Design review of the part built by this model. Coordinates are the model's own, in mm. A direction names the side the tool comes from. Give positions to 0.01 mm unless a question says otherwise; leave off trailing zeros. Loops run counter-clockwise (first coordinate to the right, second up) from the corner with the lowest first, then second, coordinate; pieces in that order, holes last. Notation, with made-up numbers: M 3.5,65.25 L 17.5,65.25 A13 ccw 17.5,85.25 Z; hole C -9.5,48 d9. An arc over 180 degrees is marked long. Use CSV: the item, a comma, the result in double quotes.
from build123d import *

# Parameters (mm, degrees)
PIPESKETCH_R    = 16.764
PIPESKETCH_R_2  = 13.3858
EXTRUSION_DEPTH = 78.43305879
SKETCH_1_R      = 16.764
SKETCH_1_R_2    = 13.3858
REVOLVE_1_ANGLE = 45.819311821
SKETCH_2_R      = 16.764
SKETCH_2_R_2    = 13.3858
EXTRUDE_1_DEPTH = 197.43866419
SKETCH_3_R      = 16.764
SKETCH_3_R_2    = 13.3858
REVOLVE_2_ANGLE = 90
SKETCH_4_R      = 16.764
SKETCH_4_R_2    = 13.3858
EXTRUDE_2_DEPTH = 120.923725302


with BuildPart() as part:
    # PipeSketch → Extrusion (new body)
    with BuildSketch(Plane.XY):
        Circle(PIPESKETCH_R)
        Circle(PIPESKETCH_R_2, mode=Mode.SUBTRACT)
    extrude(amount=EXTRUSION_DEPTH)

    # 草图1 → 旋转1 (revolve)
    with BuildSketch(Plane.XY.offset(78.43305879)):
        with Locations(Location((0, 0, 0), (0, 0, 40.203758457))):
            Circle(SKETCH_1_R)
        with Locations(Location((0, 0, 0), (0, 0, 40.203758457))):
            Circle(SKETCH_1_R_2, mode=Mode.SUBTRACT)
    revolve(axis=Axis((-29.09901546, -24.593846776, 78.43305879), (0.6455077894006402, -0.7637536866183356, 0)), revolution_arc=REVOLVE_1_ANGLE)

    # 草图2 → 凸台-拉伸1 (add)
    with BuildSketch(Plane(origin=(-44.905078471, -37.952783004, 57.137323745), x_dir=(0.8366600265340762, -0.3030542664308184, 0.4562434784170373), z_dir=(-0.5477225575051652, -0.4629230385328477, 0.6969234250586765))):
        with Locations(Location((43.130838557, 52.305939514, 0), (0, 0, 50.491424948))):
            Circle(SKETCH_2_R)
        with Locations(Location((43.130838557, 52.305939514, 0), (0, 0, 50.491424948))):
            Circle(SKETCH_2_R_2, mode=Mode.SUBTRACT)
    extrude(amount=EXTRUDE_1_DEPTH)

    # 草图3 → 旋转2 (revolve)
    with BuildSketch(Plane(origin=(-153.046688572, -129.351689355, 194.736953831), x_dir=(0.8366600265340762, -0.3030542664308184, 0.4562434784170373), z_dir=(-0.5477225575051652, -0.4629230385328477, 0.6969234250586765))):
        with Locations(Location((43.130838557, 52.305939514, 0), (0, 0, 310.893394649))):
            Circle(SKETCH_3_R)
        with Locations(Location((43.130838557, 52.305939514, 0), (0, 0, 310.893394649))):
            Circle(SKETCH_3_R_2, mode=Mode.SUBTRACT)
    revolve(axis=Axis((-137.829069481, -67.303204468, 247.911671562), (-0.6324555320336762, -0.31622776601683844, -0.707106781186547)), revolution_arc=REVOLVE_2_ANGLE)

    # 草图4 → 凸台-拉伸2 (add)
    with BuildSketch(Plane(origin=(-27.059582229, 40.909884227, 5.907369706), x_dir=(0.8366600265340752, 0.5420999882976981, 0.07827900540781119), z_dir=(-0.5477225575051666, 0.8280714102029578, 0.11957315586905065))):
        with Locations(Location((-157.337165059, -283.786451217, 0), (0, 0, 229.106605351))):
            Circle(SKETCH_4_R)
        with Locations(Location((-157.337165059, -283.786451217, 0), (0, 0, 229.106605351))):
            Circle(SKETCH_4_R_2, mode=Mode.SUBTRACT)
    extrude(amount=EXTRUDE_2_DEPTH)


solid = part.part
(1) We need section B-B on y = -28. Count the separate pieces of the cut face and the enclosed holes in it, then the cut area to 3 significant figures.
A:
separate pieces,"2"
enclosed holes,"2"
area,"1,080 mm²"
(2) We need section A-A on z = 65. State the section outline as (x, y) points.
A:
outline,"C 0,0 d33.53; hole C 0,0 d26.77"
(3) Clearance check with flat-ended pins moving along their axes: P1, Ø24, axis at x = 0, y = 0, coming from the +Z side; P2, Ø12, axis at x = -175, y = -68.5, coming from the -Z side; P3, Ø2, axis at y = -93, z = 271.5, coming from the +X side. State where each tip first meets the part, or that it passes through.
A:
P1,"z = 129.57"
P2,"z = 259.76"
P3,"x = -124.65"
(4) The part is to be moulded in two halves that separate along Z. For faces 3 (the flat face through (-1, -14, 0)), 4 (the cylindrical face through (-187.35, -35.28, 297.87)), 5 (the cylindrical face through (-52.24, -50.87, 182.46)), 6 (the flat face through (-232.797, 11.509, 278.4)), say which applies: released by +Z, released by -Z, zero draft, split by the parting line, or undercut.
A:
face 3,"released by -Z"
face 4,"split by the parting line"
face 5,"undercut"
face 6,"released by +Z"
(5) Machinability: for faces 1 (the cylindrical face through (-190.68, -33.23, 268.43)), 2 (the cylindrical face through (6.177, -11.876, 38.667)), which of the approach directions +Z, -Z, +X, -X, +Y, -Y give a long, thin tool a straight path to every point of the face, cutting with its end or side? Answer none if there is none.
A:
face 1,"none"
face 2,"-Z"
(6) Wall thickness on line 1 along Y through (x, z) = (0, 55); line 2 along Y through (x, z) = (-41.5, 158.5): over which ranges is each line inside the solid? List them lowest first. Write a range as [from, to].
A:
line 1,"[-16.76, -13.39], [13.39, 16.76]"
line 2,"[-56.9, -52.6], [-26.71, -22.42]"
